Read the model definition and answer for the solid it produces. Units are mm, in the model's axes. Face numbers are marked on the shaded views. Round coordinates to 2 decimals unless told otherwise and drop trailing zeros. Order: outer loops, then holes, each group sorted by start corner. A loop starts at its lowest first (then second) coordinate and runs counter-clockwise, first axis right, second up.
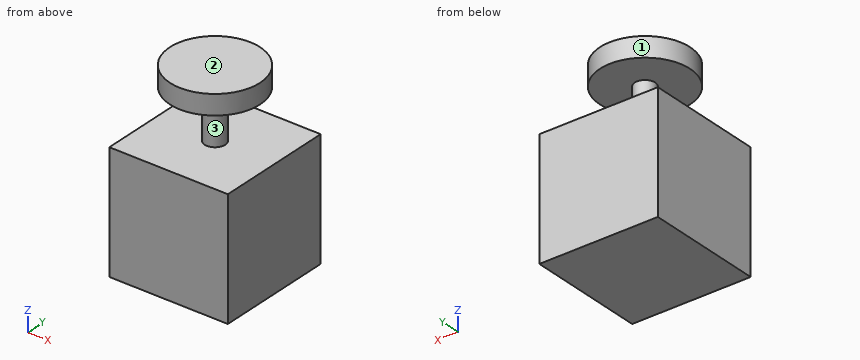
from build123d import *

# Parameters (mm, degrees)
F0_W     = 60
F0_H     = 60
F1_DEPTH = 60
F2_R     = 5.197048
F3_DEPTH = 25
F4_R     = 22.808201
F5_DEPTH = 10


with BuildPart() as f1:
    # F0 (on Top) → F1 (new body)
    with BuildSketch(Plane.XY):
        Rectangle(F0_W, F0_H)
    extrude(amount=F1_DEPTH)

    # F2 (on face) → F3 (join)
    with BuildSketch(Plane.XY.offset(60)):
        Circle(F2_R)
    extrude(amount=F3_DEPTH)

    # F4 (on face) → F5 (join)
    with BuildSketch(Plane.XY.offset(85)):
        Circle(F4_R)
    extrude(amount=F5_DEPTH)


solid = f1.part
Q1. A cutting plane is placed at A-A, the plane y = -8. Give the vertices of the cut face in (x, z), plus the area to 3 significant figures.
Outcome:
outline: (-30, 0) - (30, 0) - (30, 60) - (-30, 60) - close; (-21.36, 85) - (21.36, 85) - (21.36, 95) - (-21.36, 95) - close
area: 4,030 mm2
Q2. For a pull along Z with two mould halves and no side action, classify the marked faces 1, 2 and 3 as released by +Z, released by -Z, zero draft, split by the parting line, or undercut.
Outcome:
face 1: zero draft
face 2: released by +Z
face 3: undercut
Q3. A cutting plane is placed at C-C, the plane x = -4. Give the vertices of the cut face in (y, z), plus the area to 4 significant figures.
Outcome:
outline: (-30, 0) - (30, 0) - (30, 60) - (3.32, 60) - (3.32, 85) - (22.45, 85) - (22.45, 95) - (-22.45, 95) - (-22.45, 85) - (-3.32, 85) - (-3.32, 60) - (-30, 60) - close
area: 4,215 mm2
Q4. A cutting plane is placed at D-D, the plane y = 0. Give the vertices of the cut face in (x, z), plus the area to 3 significant figures.
Outcome:
outline: (-30, 0) - (30, 0) - (30, 60) - (5.2, 60) - (5.2, 85) - (22.81, 85) - (22.81, 95) - (-22.81, 95) - (-22.81, 85) - (-5.2, 85) - (-5.2, 60) - (-30, 60) - close
area: 4,320 mm2
Q5. Straight lines are drawn through the part: probe 1 along Z at (x, y) = (-6, 6.5); probe 2 along Z at (x, y) = (25.5, -6.5); probe 3 along Y at (x, z) = (0, 78). For each, find the intervals that lie inside material, in ascending order.
Outcome:
probe 1: z = 0 to 60, 85 to 95
probe 2: z = 0 to 60
probe 3: y = -5.2 to 5.2
Q6. A cutting plane is placed at B-B, the plane x = 7. Give the vertices of the cut face in (y, z), plus the area to 3 significant figures.
Outcome:
outline: (-30, 0) - (30, 0) - (30, 60) - (-30, 60) - close; (-21.71, 85) - (21.71, 85) - (21.71, 95) - (-21.71, 95) - close
area: 4,030 mm2
